Geometry check sheet. Reference: drawing and pictorial views, mm from the part's lowest x, y, z. A direction names the side the tool comes from. Give positions to 0.01 mm unless a question says otherwise; leave off trailing zeros. Loops run counter-clockwise (first coordinate to the right, second up) from the corner with the lowest first, then second, coordinate; pieces in that order, holes last. Notation, with made-up numbers: M -16,8.25 L 35,8.25 A14 ccw 35,23.25 Z; hole C 28,81.5 d6. An arc over 180 degrees is marked long. Use CSV: the item, a comma, the result in double quotes.
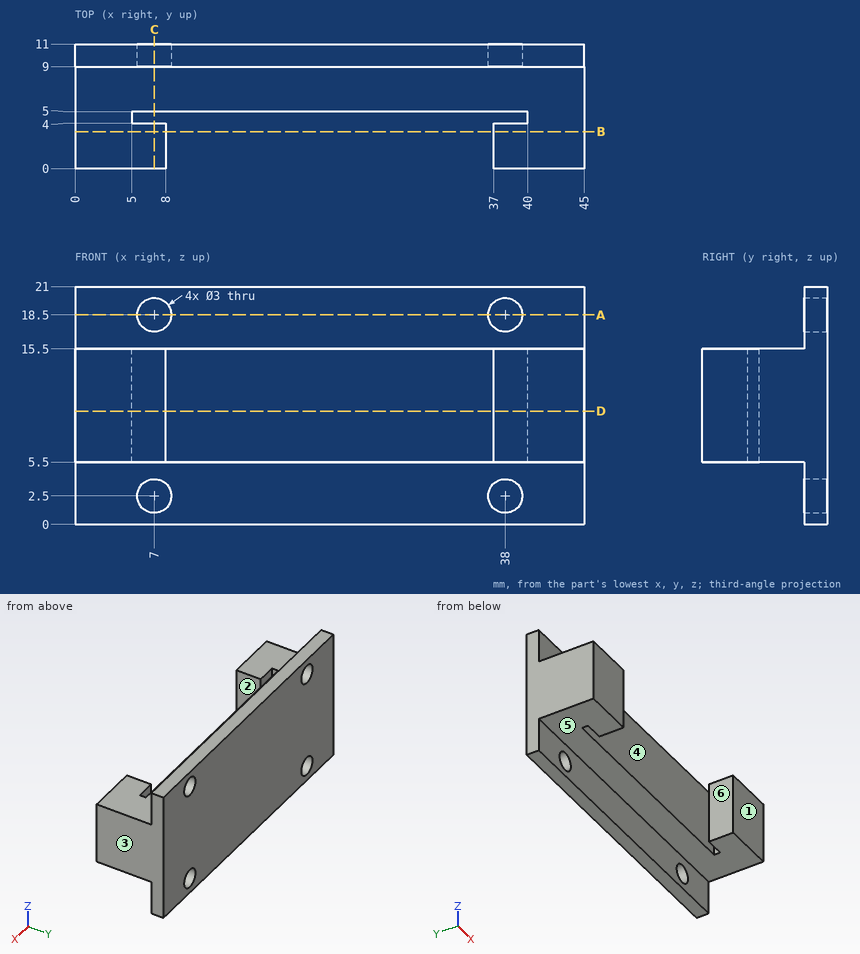
(1) Depth check by flat-ended pin: pin 1 Ø0.5 at (y, z) = (4.5, 12.5) entering from -X; pin 2 Ø4 at (x, z) = (7, 2.5) entering from -Y; pin 3 Ø4.5 at (x, z) = (25.5, 4) entering from -Y; pin 4 Ø1.5 at (x, y) = (7.5, 6) entering from -Z. Enter the tip coordinate at first touch or a pass-through.
Calculated:
pin 1,"stops at x = 0"
pin 2,"stops at y = 9"
pin 3,"stops at y = 5"
pin 4,"stops at z = 5.5"
(2) Scan lines: L1, parallel to Z at x = 38, y = 9.6; L2, parallel to X at y = 10.3, z = 18.5; L3, parallel to X at y = 9.5, z = 1.75. Record each from-to range of solid material in increasing order. Write a range as from..to.
Calculated:
L1,"z = 0..1, 4..17, 20..21"
L2,"x = 0..5.5, 8.5..36.5, 39.5..45"
L3,"x = 0..5.7, 8.3..36.7, 39.3..45"
(3) Section check C-C on x = 7. Record the cut outline in (y, z), plus the area to 3 significant figures.
Calculated:
outline,"M 0,5.5 L 4,5.5 L 4,15.5 L 0,15.5 Z; M 5,5.5 L 9,5.5 L 9,4 L 11,4 L 11,17 L 9,17 L 9,15.5 L 5,15.5 Z; M 9,0 L 11,0 L 11,1 L 9,1 Z; M 9,20 L 11,20 L 11,21 L 9,21 Z"
area,"110 mm²"
(4) Mould release check, pull along X, two halves, no side actions. Record for the marked faces 1, 2 and 3: released by +X, released by -X, zero draft, split by the parting line, or undercut.
Calculated:
face 1,"zero draft"
face 2,"undercut"
face 3,"released by +X"
(5) Section check B-B on y = 3.25. Record the cut outline in (x, z).
Calculated:
outline,"M 0,5.5 L 8,5.5 L 8,15.5 L 0,15.5 Z; M 37,5.5 L 45,5.5 L 45,15.5 L 37,15.5 Z"
(6) Section check A-A on z = 18.5. Record the cut outline in (x, y), plus the area to 3 significant figures.
Calculated:
outline,"M 0,9 L 5.5,9 L 5.5,11 L 0,11 Z; M 8.5,9 L 36.5,9 L 36.5,11 L 8.5,11 Z; M 39.5,9 L 45,9 L 45,11 L 39.5,11 Z"
area,"78.0 mm²"
(7) Tool access check on the marked faces 4, 5 and 6. Record the directions out of +Z, -Z, +X, -X, +Y, -Y that give a thin tool (end or side, any length) a straight path to the whole face; none if there is none.
Calculated:
face 4,"+Z, -Z"
face 5,"-Z, +X, -X, -Y"
face 6,"+Z, -Z, -Y"
(8) Section check D-D on z = 10. Record the cut outline in (x, y), plus the area to 3 significant figures.
Calculated:
outline,"M 0,0 L 8,0 L 8,4 L 5,4 L 5,5 L 40,5 L 40,4 L 37,4 L 37,0 L 45,0 L 45,11 L 0,11 Z"
area,"344 mm²"
